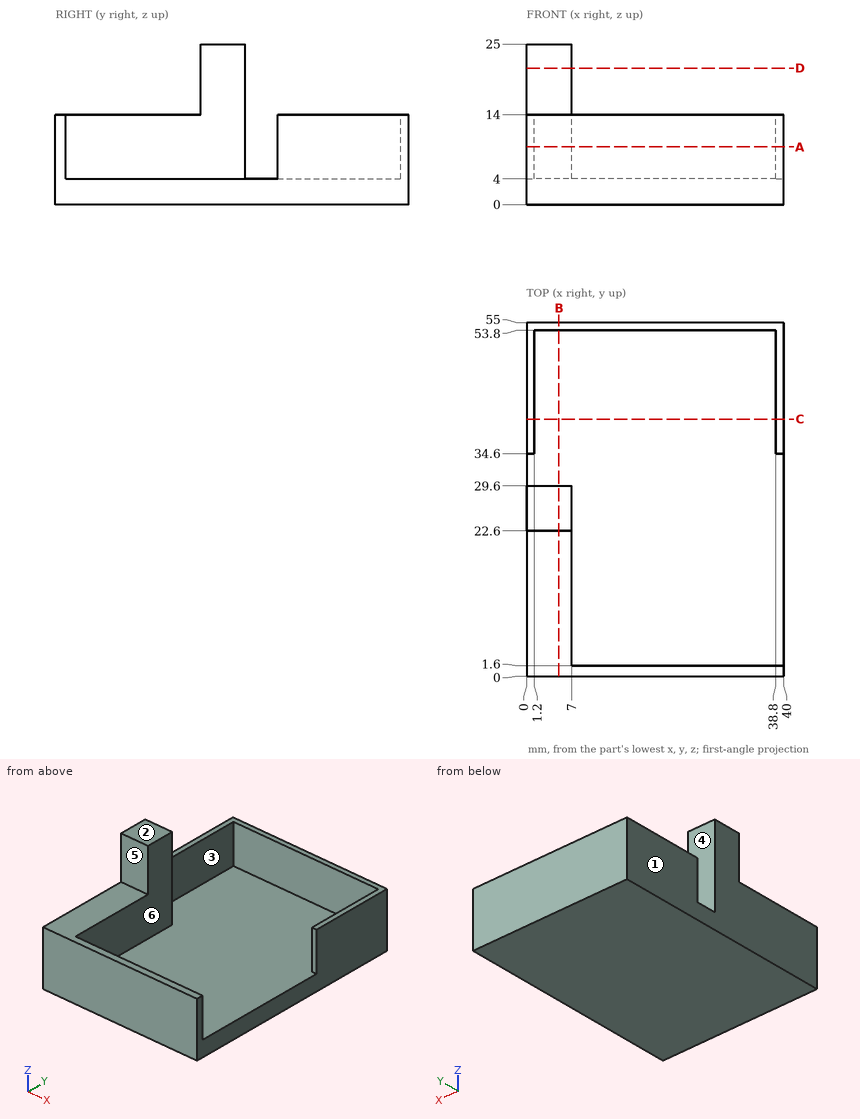
Design review of the part shown in the three views and the two pictorial views. Dimensions are in mm from the part's minimum x, y and z. A direction names the side the tool comes from. Coordinates: 2 decimals unless noted, no trailing zeros. Loops run counter-clockwise (first coordinate to the right, second up) from the corner with the lowest first, then second, coordinate; pieces in that order, holes last. Notation, with made-up numbers: (40.5, 9.25) - (70.5, 9.25) arc R20 ccw to (70.5, 20.25) - close; hole circle Ø11 at (2, 48). An arc over 180 degrees is marked (long way). Use a Markdown table: item, result. Add a question column.
Item 1: Insertion check: pin 1 Ø8 at (y, z) = (42.5, 8) entering from -X; pin 2 Ø5.5 at (x, z) = (2.5, 18) entering from -Y; pin 3 Ø6 at (x, y) = (5, 40.5) entering from +Z; pin 4 Ø18 at (x, y) = (14.5, 15.5) entering from +Z. Each pin has a flat end and moves straight along its axis. Give the tip position at first contact, or say it passes through.
Item 2: We need section B-B (x = 5). Give the boundary of the cut face in (y, z).
Item 3: We need section A-A (z = 9). Give the boundary of the cut face in (x, y).
Item 4: Tool access review of the marked faces 4, 5 and 6: name each direction out of +Z, -Z, +X, -X, +Y, -Y from which nothing blocks a thin tool from reaching the whole face with its end or side.
Item 5: For line 1 (X direction, y = 46, z = 13.5); line 2 (Y direction, x = 24, z = 4.25); line 3 (Z direction, x = 26, y = 11.5), list the stretches that pass through material, from the lowest coordinate up.
Item 6: Mouldability with a two-part tool opening along X and no side actions: class the marked faces 1, 2 and 3 as pulls with the +X half, pulls with the -X half, needs draft (parallel to the pull), parting line crosses it, or undercut.
Item 7: We need section C-C (y = 40). Give the boundary of the cut face in (x, z), and give its area (3 significant figures).
Item 8: We need section D-D (z = 21.25). Give the boundary of the cut face in (x, y).
Results list:
| question | item | result |
|---|---|---|
| 1 | pin 1 | stops at x = 0 |
| 1 | pin 2 | stops at y = 22.6 |
| 1 | pin 3 | stops at z = 4 |
| 1 | pin 4 | stops at z = 14 |
| 2 | outline | (0, 0) - (55, 0) - (55, 14) - (53.8, 14) - (53.8, 4) - (29.6, 4) - (29.6, 25) - (22.6, 25) - (22.6, 14) - (0, 14) - close |
| 3 | outline | (0, 0) - (40, 0) - (40, 1.6) - (7, 1.6) - (7, 29.6) - (0, 29.6) - close; (0, 34.6) - (1.2, 34.6) - (1.2, 53.8) - (38.8, 53.8) - (38.8, 34.6) - (40, 34.6) - (40, 55) - (0, 55) - close |
| 4 | face 4 | +Z, +X, -X |
| 4 | face 5 | +Z, +X, -X, -Y |
| 4 | face 6 | +Z, +X |
| 5 | line 1 | x = 0 to 1.2, 38.8 to 40 |
| 5 | line 2 | y = 0 to 1.6, 53.8 to 55 |
| 5 | line 3 | z = 0 to 4 |
| 6 | face 1 | pulls with the -X half |
| 6 | face 2 | needs draft |
| 6 | face 3 | undercut |
| 7 | outline | (0, 0) - (40, 0) - (40, 14) - (38.8, 14) - (38.8, 4) - (1.2, 4) - (1.2, 14) - (0, 14) - close |
| 7 | area | 184 mm^2 |
| 8 | outline | (0, 22.6) - (7, 22.6) - (7, 29.6) - (0, 29.6) - close |
